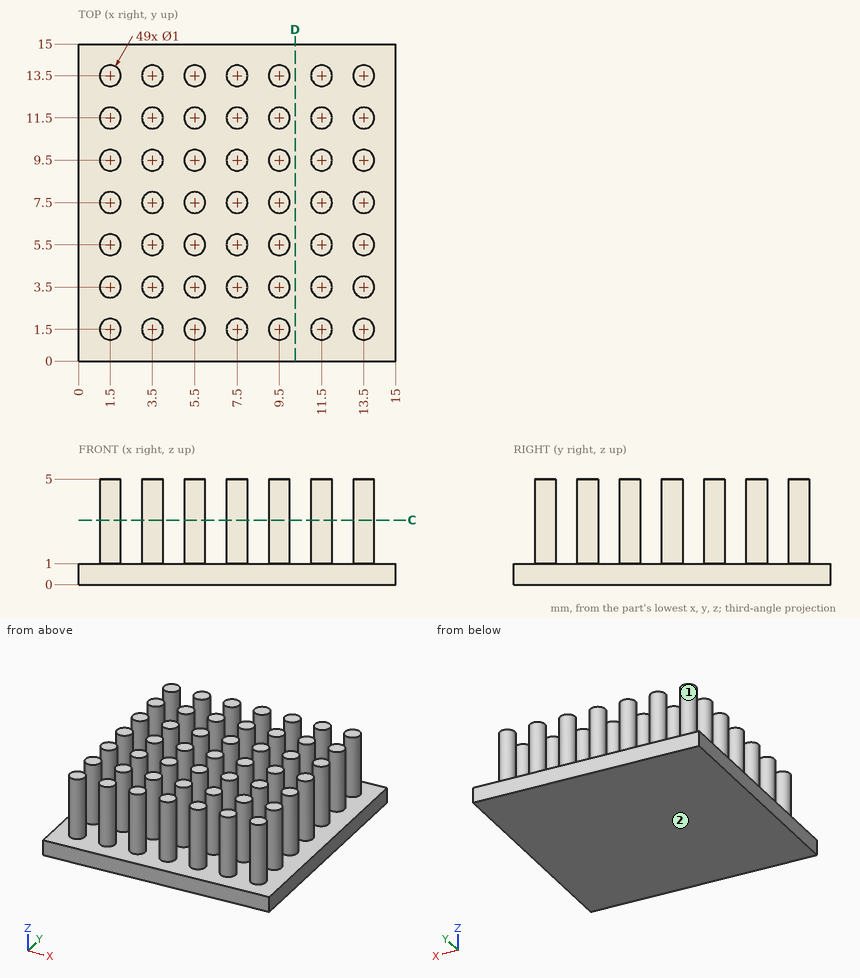
Check sheet for the drawn part. Datum: minimum x, y, z corner. Units: mm. Coordinates: 2 decimals unless noted, no trailing zeros. Order: outer loops, then holes, each group sorted by start corner. A loop starts at its lowest first (then second) coordinate and runs counter-clockwise, first axis right, second up. Notation, with made-up numbers: M 54.25,44.5 L 82.25,44.5 A13 cw 82.25,66.5 Z; hole C 89.25,35 d10. An arc over 180 degrees is marked long. One line per item, written item: value. Start each with the question number.
Item 1: Sectioned sample at D-D (x = 10.25). Enter the section's corners in (y, z), then the cut area to 3 significant figures.
Item 2: Gauge pin test, flat end, axial feed: pin 1 (2 mm diameter, centred on x = 11, z = 3, fed in from +Y). Record the tip position at first contact, or that the pin passes through.
Item 3: Sectioned sample at C-C (z = 3.05). Count the separate pieces of the cut face and the enclosed holes in it, then the cut area to 3 significant figures.
Item 4: Mould release check, pull along Y, two halves, no side actions. Record for the marked faces 1 and 2: released by +Y, released by -Y, zero draft, split by the parting line, or undercut.
Item 5: Scan line: probe 1 along Z at (x, y) = (10, 9.25). Record every from-to range of solid material in increasing order.
Conclusion:
1. outline: M 0,0 L 15,0 L 15,1 L 0,1 Z
1. area: 15.0 mm^2
2. pin 1: stops at y = 14
3. separate pieces: 49
3. enclosed holes: 0
3. area: 38.5 mm^2
4. face 1: undercut
4. face 2: zero draft
5. probe 1: z = 0 to 1
